Design review of the part shown in the three views and the two pictorial views. Dimensions are in mm from the part's minimum x, y and z. A direction names the side the tool comes from. Give positions to 0.01 mm unless a question says otherwise; leave off trailing zeros. Order: outer loops, then holes, each group sorted by start corner. A loop starts at its lowest first (then second) coordinate and runs counter-clockwise, first axis right, second up. Notation, with made-up numbers: M 59.5,79 L 115.5,79 A10 ccw 115.5,85 Z; hole C 8.25,23 d4. An arc over 180 degrees is marked long. Answer as a JSON object with one key per item and string values.
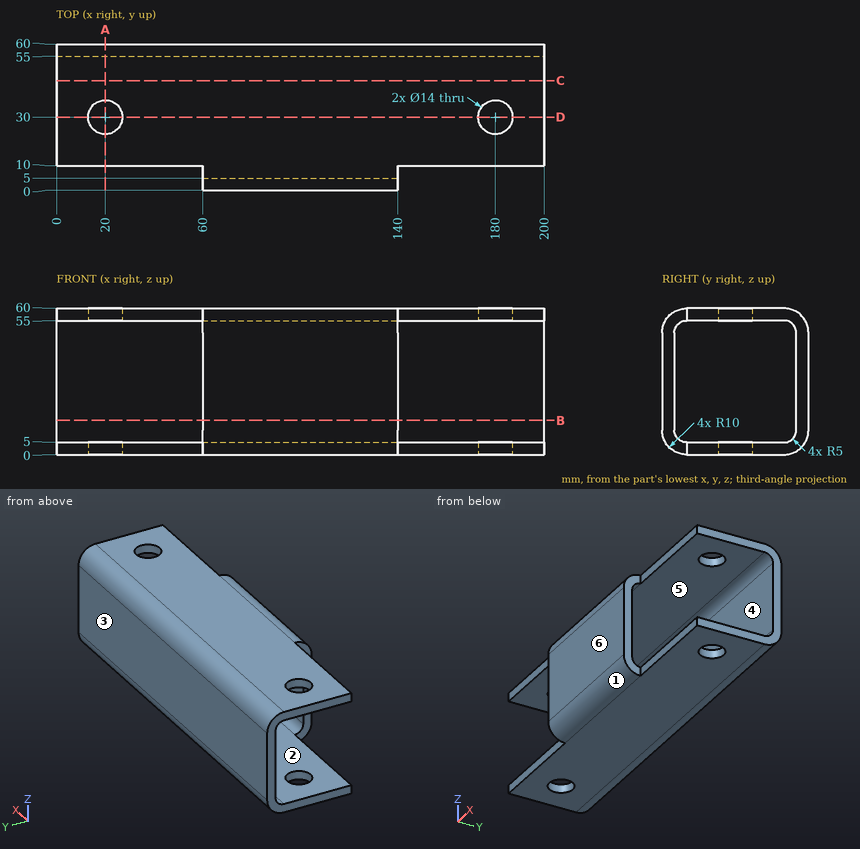
(1) We need section C-C (y = 45). Write out the cut boundary in (x, z), plus the area to 3 significant figures.
Checked values:
{"outline": "M 0,0 L 200,0 L 200,5 L 0,5 Z; M 0,55 L 200,55 L 200,60 L 0,60 Z", "area": "2,000 mm^2"}
(2) We need section A-A (x = 20). Write out the cut boundary in (y, z), plus the area to 3 significant figures.
Checked values:
{"outline": "M 10,0 L 23,0 L 23,5 L 10,5 Z; M 10,55 L 23,55 L 23,60 L 10,60 Z; M 37,0 L 50,0 A10 ccw 60,10 L 60,50 A10 ccw 50,60 L 37,60 L 37,55 L 50,55 A5 cw 55,50 L 55,10 A5 cw 50,5 L 37,5 Z", "area": "578 mm^2"}
(3) Insertion check: pin 1 (1.5 mm diameter, centred on x = 19.5, z = 56.5, fed in from -Y); pin 2 (3 mm diameter, centred on y = 3, z = 44, fed in from +X); pin 3 (2 mm diameter, centred on x = 107, y = 6, fed in from +Z). Each pin has a flat end and moves straight along its axis. Give the tip position at first contact, or say it passes through.
Checked values:
{"pin 1": "stops at y = 10", "pin 2": "stops at x = 140", "pin 3": "stops at z = 59.54"}
(4) Draft analysis for pull direction Y (two halves, no side actions). For the marked faces 3, 4, 5 and 6, state which applies: +Y half, -Y half, draft (parallel to the pull), parting line (faces both ways), or undercut.
Checked values:
{"face 3": "+Y half", "face 4": "undercut", "face 5": "undercut", "face 6": "-Y half"}
(5) Tool access review of the marked faces 1 and 2: name each direction out of +Z, -Z, +X, -X, +Y, -Y from which nothing blocks a thin tool from reaching the whole face with its end or side.
Checked values:
{"face 1": "-Z, +X, -X, -Y", "face 2": "+X, -X"}
(6) To check wall thickness, follow L1, parallel to Z at x = 54, y = 15; L2, parallel to Y at x = 159.5, z = 23.5. State the ranges of each line that lie inside material, in increasing order. Write a range as from..to.
Checked values:
{"L1": "z = 0..5, 55..60", "L2": "y = 55..60"}
(7) We need section B-B (z = 14). Write out the cut boundary in (x, y).
Checked values:
{"outline": "M 0,55 L 200,55 L 200,60 L 0,60 Z; M 60,0 L 140,0 L 140,5 L 60,5 Z"}
(8) We need section D-D (y = 30). Write out the cut boundary in (x, z).
Checked values:
{"outline": "M 0,0 L 13,0 L 13,5 L 0,5 Z; M 0,55 L 13,55 L 13,60 L 0,60 Z; M 27,0 L 173,0 L 173,5 L 27,5 Z; M 27,55 L 173,55 L 173,60 L 27,60 Z; M 187,0 L 200,0 L 200,5 L 187,5 Z; M 187,55 L 200,55 L 200,60 L 187,60 Z"}
